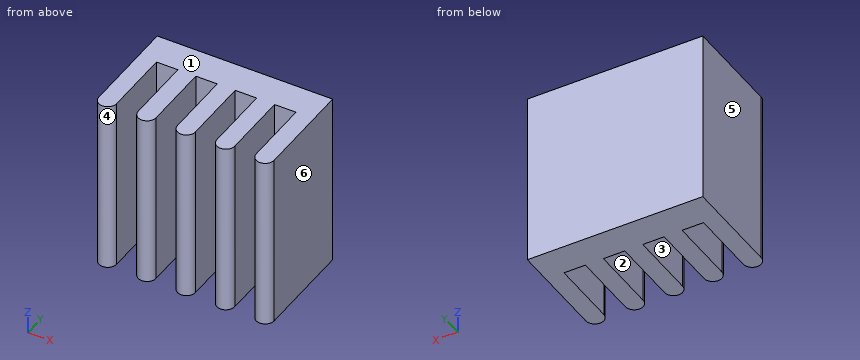
```python
from build123d import *

# Parameters (mm, degrees)
RESSALTO_EXTRUS_O1_DEPTH = 4.4


with BuildPart() as part:
    # Esboço1 → Ressalto-extrusão1 (new body, symmetric)
    with BuildSketch(Plane.XY):
        with BuildLine():
            Line((0, 0), (8.8, 0))
            Line((8.8, 0), (8.8, -5))
            ThreePointArc((8.8, -5), (8.35, -5.45), (7.9, -5))
            Line((7.9, -5), (7.9, -1.6))
            Line((7.9, -1.6), (6.825, -1.6))
            Line((6.825, -1.6), (6.825, -5))
            ThreePointArc((6.825, -5), (6.375, -5.45), (5.925, -5))
            Line((5.925, -5), (5.925, -1.6))
            Line((5.925, -1.6), (4.85, -1.6))
            Line((4.85, -1.6), (4.85, -5))
            ThreePointArc((4.85, -5), (4.4, -5.45), (3.95, -5))
            Line((3.95, -5), (3.95, -1.6))
            Line((3.95, -1.6), (2.875, -1.6))
            Line((2.875, -1.6), (2.875, -5))
            ThreePointArc((2.875, -5), (2.425, -5.45), (1.975, -5))
            Line((1.975, -5), (1.975, -1.6))
            Line((1.975, -1.6), (0.9, -1.6))
            Line((0.9, -1.6), (0.9, -5))
            ThreePointArc((0.9, -5), (0.45, -5.45), (0, -5))
            Line((0, -5), (0, 0))
        make_face()
    extrude(amount=RESSALTO_EXTRUS_O1_DEPTH, both=True)


solid = part.part
```
Design review of the part built by this model. Coordinates are the model's own, in mm. Face numbers are marked on the shaded views. A direction names the side the tool comes from. Coordinates: 2 decimals unless noted, no trailing zeros. Order: outer loops, then holes, each group sorted by start corner. A loop starts at its lowest first (then second) coordinate and runs counter-clockwise, first axis right, second up. Notation, with made-up numbers: (16, 9.5) - (74, 9.5) arc R25 ccw to (74, 30.5) - close; hole circle Ø2 at (-20.75, -28). An arc over 180 degrees is marked (long way). Answer in a Markdown table with one row per item.
(1) Clearance check with a flat-ended pin moving along its axis: pin 1 (1 mm diameter, centred on x = 1, z = 1, fed in from +Y). State where the tip first meets the part, or that it passes through.
Checked values:
| item | result |
|---|---|
| pin 1 | y = 0 |
(2) Consider section C-C on x = 7.75. State the section outline as (y, z) points.
Checked values:
| item | result |
|---|---|
| outline | (-1.6, -4.4) - (0, -4.4) - (0, 4.4) - (-1.6, 4.4) - close |
(3) For the marked faces 1 and 2, list the 3-axis set-ups (+Z, -Z, +X, -X, +Y, -Y) from which the entire face can be reached by the end or side of a thin tool; tool diameter is ignored.
Checked values:
| item | result |
|---|---|
| face 1 | +Z, +X, -X, +Y, -Y |
| face 2 | +Z, -Z, -Y |
(4) Consider section A-A on y = -2.9. State the section outline as (x, z) points (3 decimals).
Checked values:
| item | result |
|---|---|
| outline | (0, -4.4) - (0.9, -4.4) - (0.9, 4.4) - (0, 4.4) - close; (1.975, -4.4) - (2.875, -4.4) - (2.875, 4.4) - (1.975, 4.4) - close; (3.95, -4.4) - (4.85, -4.4) - (4.85, 4.4) - (3.95, 4.4) - close; (5.925, -4.4) - (6.825, -4.4) - (6.825, 4.4) - (5.925, 4.4) - close; (7.9, -4.4) - (8.8, -4.4) - (8.8, 4.4) - (7.9, 4.4) - close |
(5) Consider section B-B on z = 2.75. State the section outline as (x, y) points (3 decimals), plus the area to 3 significant figures.
Checked values:
| item | result |
|---|---|
| outline | (0, -5) arc R0.45 ccw to (0.9, -5) - (0.9, -1.6) - (1.975, -1.6) - (1.975, -5) arc R0.45 ccw to (2.875, -5) - (2.875, -1.6) - (3.95, -1.6) - (3.95, -5) arc R0.45 ccw to (4.85, -5) - (4.85, -1.6) - (5.925, -1.6) - (5.925, -5) arc R0.45 ccw to (6.825, -5) - (6.825, -1.6) - (7.9, -1.6) - (7.9, -5) arc R0.45 ccw to (8.8, -5) - (8.8, 0) - (0, 0) - close |
| area | 31.0 mm^2 |
(6) The part is to be moulded in two halves that separate along X. For the marked faces 3, 4, 5 and 6, say which applies: released by +X, released by -X, zero draft, split by the parting line, or undercut.
Checked values:
| item | result |
|---|---|
| face 3 | undercut |
| face 4 | undercut |
| face 5 | released by -X |
| face 6 | released by +X |
(7) Wall thickness on line 1 along X through (y, z) = (-4.3, -2.5) (3 decimals); line 2 along Y through (x, z) = (0.5, 0); line 3 along Y through (x, z) = (7, -2.75): over which ranges is each line inside the solid? List them lowest first. Write a range as from..to.
Checked values:
| item | result |
|---|---|
| line 1 | 0..0.9, 1.975..2.875, 3.95..4.85, 5.925..6.825, 7.9..8.8 |
| line 2 | -5.45..0 |
| line 3 | -1.6..0 |
